Design review of the part shown in the three views and the two pictorial views. Dimensions are in mm from the part's minimum x, y and z. A direction names the side the tool comes from. Coordinates: 2 decimals unless noted, no trailing zeros. Order: outer loops, then holes, each group sorted by start corner. A loop starts at its lowest first (then second) coordinate and runs counter-clockwise, first axis right, second up. Notation, with made-up numbers: (31.5, -18) -> (62.5, -18) arc R25 ccw to (62.5, -6) -> close; hole circle Ø11 at (37, -35.5). An arc over 180 degrees is marked (long way). Answer as a JSON object with one key per item and string values. Group by question number.
1) Add section A-A, the plane z = 10. Write out the cut boundary in (x, y).
2) Add section D-D, the plane y = 10.5. Write out the cut boundary in (x, z).
3) Add section C-C, the plane x = 4. Write out the cut boundary in (y, z).
4) Machinability: for the marked faces 1 and 2, which of the approach directions +Z, -Z, +X, -X, +Y, -Y give a long, thin tool a straight path to every point of the face, cutting with its end or side? Answer none if there is none.
5) Add section B-B, the plane x = 24. Write out the cut boundary in (y, z), then the cut area to 3 significant figures.
6) Wall thickness on L1, parallel to X at y = 1.2, z = 10; L2, parallel to Z at x = 24, y = 2; L3, parallel to Y at x = 16, z = 1.75: over which ranges is each line inside the solid? List them lowest first.
7) For pin 1 (3 mm diameter, centred on x = 12, z = 10, fed in from +Y); pin 2 (4 mm diameter, centred on x = 22.5, y = 49, fed in from -Z); pin 3 (4 mm diameter, centred on x = 29.5, z = 6, fed in from -Y); pin 4 (10 mm diameter, centred on x = 17, z = 5.5, fed in from +Y), all flat-tipped, find the tip position at first contact; note any pin that passes through.
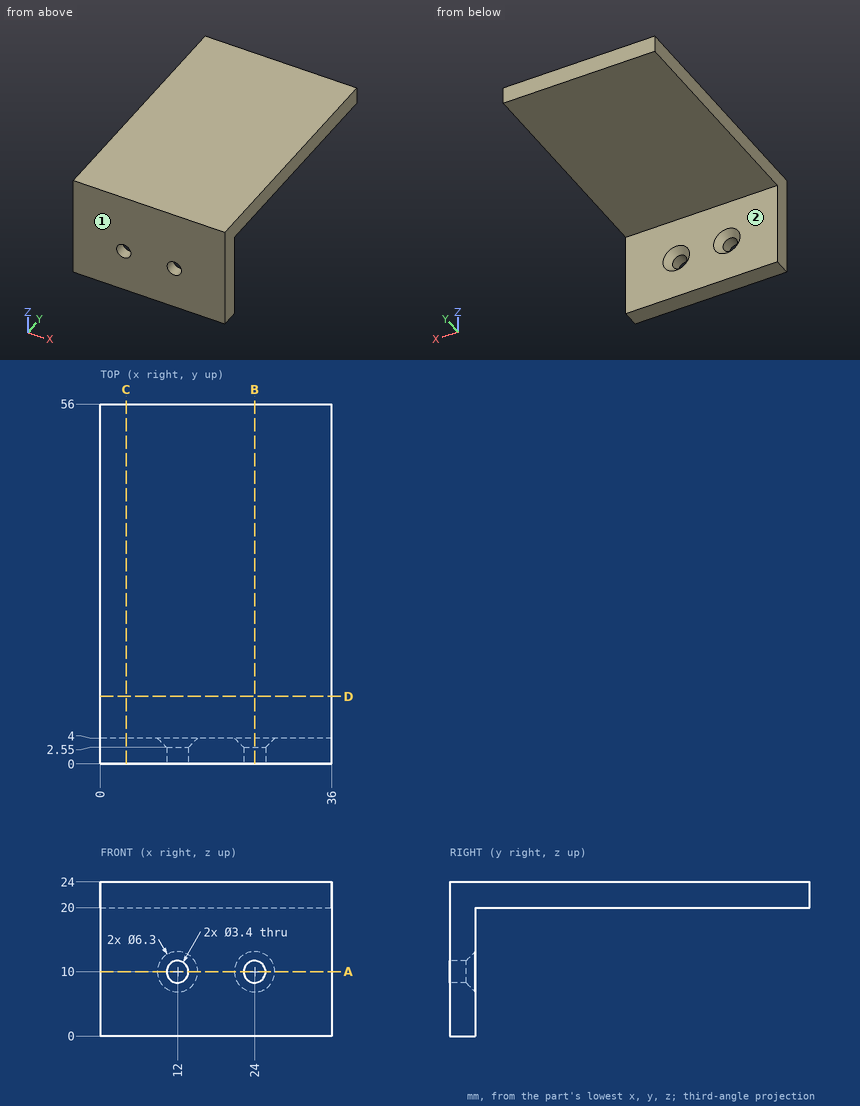
Output values:
{
 "1": {"outline": "(0, 0) -> (10.3, 0) -> (10.3, 2.55) -> (8.85, 4) -> (0, 4) -> close; (13.7, 0) -> (22.3, 0) -> (22.3, 2.55) -> (20.85, 4) -> (15.15, 4) -> (13.7, 2.55) -> close; (25.7, 0) -> (36, 0) -> (36, 4) -> (27.15, 4) -> (25.7, 2.55) -> close"},
 "2": {"outline": "(0, 20) -> (36, 20) -> (36, 24) -> (0, 24) -> close"},
 "3": {"outline": "(0, 0) -> (4, 0) -> (4, 20) -> (56, 20) -> (56, 24) -> (0, 24) -> close"},
 "4": {"face 1": "+Z, -Z, +X, -X, -Y", "face 2": "-Z, +X, -X, +Y"},
 "5": {"outline": "(0, 0) -> (4, 0) -> (4, 6.85) -> (2.55, 8.3) -> (0, 8.3) -> close; (0, 11.7) -> (2.55, 11.7) -> (4, 13.15) -> (4, 20) -> (56, 20) -> (56, 24) -> (0, 24) -> close", "area": "288 mm²"},
 "6": {"L1": "x = 0 to 10.3, 13.7 to 22.3, 25.7 to 36", "L2": "z = 0 to 8.3, 11.7 to 24", "L3": "y = 0 to 4"},
 "7": {"pin 1": "passes through", "pin 2": "stops at z = 20", "pin 3": "stops at y = 0", "pin 4": "stops at y = 4"}
}
